Could you check a few things on this model? Use its own coordinates, in mm. Face numbers are marked on the shaded views. A direction names the side the tool comes from. Coordinates: 2 decimals unless noted, no trailing zeros. Loops run counter-clockwise (first coordinate to the right, second up) from the corner with the lowest first, then second, coordinate; pieces in that order, holes last.
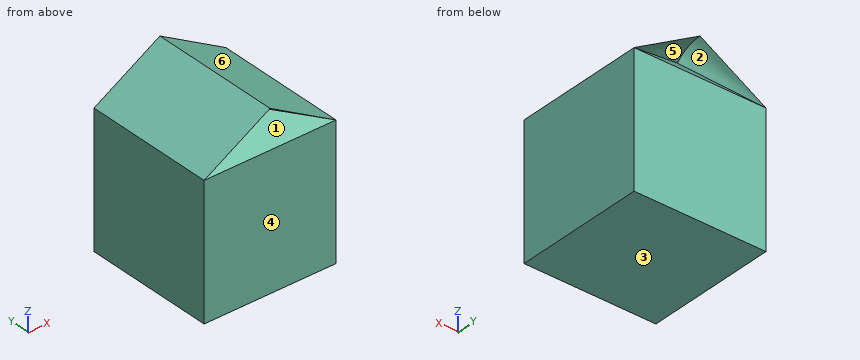
from build123d import *

# Parameters (mm, degrees)
F0_W     = 55
F0_H     = 55
F1_DEPTH = 27.5
F4_DEPTH = 27.5
F6_ANGLE = 45
F8_ANGLE = 45


with BuildPart() as f1:
    # F0 (on Front) → F1 (new body, symmetric)
    with BuildSketch(Plane.XZ):
        Rectangle(F0_W, F0_H)
    extrude(amount=F1_DEPTH, both=True)

    # F3 (on Front) → F4 (join, symmetric)
    with BuildSketch(Plane.XZ):
        Polygon((27.5, 27.5), (0, 43.5133390129), (-27.5, 27.5), align=None)
    extrude(amount=F4_DEPTH, both=True)

    # F5 (on face) → F6 (revolve, cut)
    with BuildSketch(Plane.XZ.offset(27.5)):
        Polygon((0, 43.5133390129), (-27.5, 27.5), (27.5, 27.5), align=None)
    revolve(axis=Axis((0, -27.5, 27.5), (-1, 0, 0)), revolution_arc=F6_ANGLE, mode=Mode.SUBTRACT)

    # F7 (on face) → F8 (revolve, cut)
    with BuildSketch(Plane(origin=(0, 27.5, 0), x_dir=(-1, 0, 0), z_dir=(0, 1, 0))):
        Polygon((0, 43.5133390129), (-27.5, 27.5), (27.5, 27.5), align=None)
    revolve(axis=Axis((0, 27.5, 27.5), (1, 0, 0)), revolution_arc=F8_ANGLE, mode=Mode.SUBTRACT)


solid = f1.part
(1) Imagine slicing it at A-A, the plane x = 6.5. Write out the boundary of the cut face in (y, z), and give its area (3 significant figures).
Answers:
outline: (-27.5, -27.5) - (27.5, -27.5) - (27.5, 27.5) - (18.85, 36.15) arc R12.23 cw to (27.5, 39.73) - (-27.5, 39.73) arc R12.23 cw to (-18.85, 36.15) - (-27.5, 27.5) - close
area: 3,580 mm2
(2) We'd pull the mould along Z, two halves only. Please class the marked faces 4, 5 and 6: +Z half, -Z half, draft (parallel to the pull), parting line (faces both ways), or undercut.
Answers:
face 4: draft
face 5: undercut
face 6: +Z half
(3) I need wall thicknesses on probe 1 along Z at (x, y) = (-2, 23); probe 2 along X at (y, z) = (5, 37); probe 3 along Z at (x, y) = (24.5, 19). Which ranges of each line are inside material? Lowest first, please.
Answers:
probe 1: z = -27.5 to 32, 41.65 to 42.35
probe 2: x = -11.19 to 11.19
probe 3: z = -27.5 to 29.25
(4) For pin 1 (12 mm diameter, centred on x = 13.5, y = -21, fed in from +Z); pin 2 (8 mm diameter, centred on x = -21, y = 21.5, fed in from +Z); pin 3 (4 mm diameter, centred on x = 9, y = 20.5, fed in from +Z), each with a flat end and sliding along its axis, tell me the tip position at first contact or that it passes through.
Answers:
pin 1: stops at z = 39.15
pin 2: stops at z = 33.61
pin 3: stops at z = 39.44
(5) Imagine slicing it at C-C, the plane x = -12. Write out the boundary of the cut face in (y, z).
Answers:
outline: (-27.5, -27.5) - (27.5, -27.5) - (27.5, 27.5) - (21.12, 33.88) arc R9.03 cw to (27.5, 36.53) - (-27.5, 36.53) arc R9.03 cw to (-21.12, 33.88) - (-27.5, 27.5) - close
(6) Which directions (+Z, -Z, +X, -X, +Y, -Y) give clear straight access to the entire face, cutting with the end or side of a thin tool? Please do the marked faces 1, 2 and 3.
Answers:
face 1: -Y
face 2: +Y
face 3: -Z, +X, -X, +Y, -Y
(7) Imagine slicing it at B-B, the plane y = -12.5. Write out the boundary of the cut face in (x, z), and give its area (3 significant figures).
Answers:
outline: (-27.5, -27.5) - (27.5, -27.5) - (27.5, 27.5) - (0, 43.51) - (-27.5, 27.5) - close
area: 3,470 mm2
